from build123d import *

# Parameters (mm, degrees)
F0_W     = 42
F0_H     = 42
F1_DEPTH = 4
F3_R     = 5
F4_R     = 2.5
F5_DEPTH = 25


with BuildPart() as f1:
    # F0 (on Top) → F1 (new body)
    with BuildSketch(Plane.XY):
        Rectangle(F0_W, F0_H)
    extrude(amount=F1_DEPTH)

    # F3
    f3_edges = [f1.edges().sort_by_distance(p)[0] for p in [
        (-21, 21, 2),
        (-21, -21, 2),
        (21, -21, 2),
        (21, 21, 2),
    ]]
    fillet(f3_edges, radius=F3_R)

    # F4 (on face) → F5 (cut)
    with BuildSketch(Plane.XY.offset(4)):
        Circle(F4_R)
    extrude(amount=-F5_DEPTH, mode=Mode.SUBTRACT)


solid = f1.part
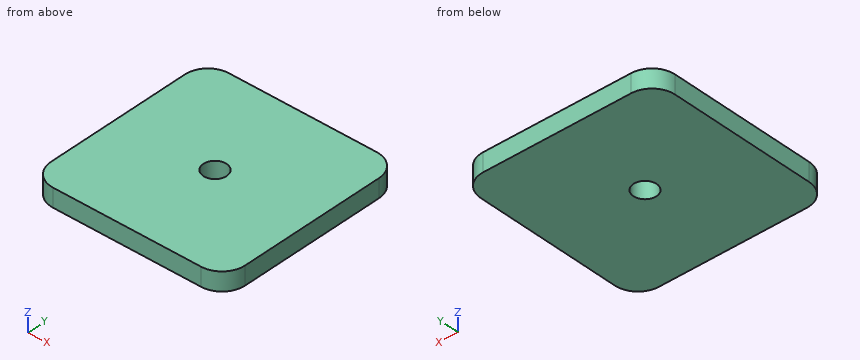
Input: part model. Units: mm. Frame: model coordinates. Give positions to 0.01 mm unless a question says otherwise; leave off trailing zeros. Order: outer loops, then holes, each group sorted by start corner. A loop starts at its lowest first (then second) coordinate and runs counter-clockwise, first axis right, second up.
Q1. Section C-C on z = 1.15. Output: boundary loops of the cut face in (x, y), and give its area (3 significant figures).
Checked values:
outline: (-21, -16) arc R5 ccw to (-16, -21) - (16, -21) arc R5 ccw to (21, -16) - (21, 16) arc R5 ccw to (16, 21) - (-16, 21) arc R5 ccw to (-21, 16) - close; hole circle Ø5 at (0, 0)
area: 1,720 mm2
Q2. Section A-A on x = 0. Output: boundary loops of the cut face in (y, z), and give its area (3 significant figures).
Checked values:
outline: (-21, 0) - (-2.5, 0) - (-2.5, 4) - (-21, 4) - close; (2.5, 0) - (21, 0) - (21, 4) - (2.5, 4) - close
area: 148 mm2
Q3. Section D-D on x = 18.5. Output: boundary loops of the cut face in (y, z).
Checked values:
outline: (-20.33, 0) - (20.33, 0) - (20.33, 4) - (-20.33, 4) - close
Q4. Ray query, probe 1 along Y at (x, z) = (0, 2.5); probe 2 along X at (y, z) = (0.5, 2); probe 3 along X at (y, z) = (-2, 2.55). Return the intervals inside material, ascending.
Checked values:
probe 1: y = -21 to -2.5, 2.5 to 21
probe 2: x = -21 to -2.45, 2.45 to 21
probe 3: x = -21 to -1.5, 1.5 to 21
